```python
from build123d import *

# Parameters (mm, degrees)
F0_W     = 355.6
F0_H     = 203.2
F0_R     = 1.25
F0_R_2   = 20.6375
F1_DEPTH = 2.54


with BuildPart() as f1:
    # F0 (on Front) → F1 (new body)
    with BuildSketch(Plane.XZ):
        with Locations((177.8, 101.6)):
            Rectangle(F0_W, F0_H)
        with BuildLine():
            Line((26.67, 62.23), (41.91, 62.23))
            ThreePointArc((41.91, 62.23), (42.808026, 61.858026), (43.18, 60.96))
            Line((43.18, 60.96), (43.18, 45.72))
            ThreePointArc((43.18, 45.72), (42.808026, 44.821974), (41.91, 44.45))
            Line((41.91, 44.45), (26.67, 44.45))
            ThreePointArc((26.67, 44.45), (25.771974, 44.821974), (25.4, 45.72))
            Line((25.4, 45.72), (25.4, 60.96))
            ThreePointArc((25.4, 60.96), (25.771974, 61.858026), (26.67, 62.23))
        make_face(mode=Mode.SUBTRACT)
        with BuildLine():
            Line((48.26, 62.23), (63.5, 62.23))
            ThreePointArc((63.5, 62.23), (64.398026, 61.858026), (64.77, 60.96))
            Line((64.77, 60.96), (64.77, 45.72))
            ThreePointArc((64.77, 45.72), (64.398026, 44.821974), (63.5, 44.45))
            Line((63.5, 44.45), (48.26, 44.45))
            ThreePointArc((48.26, 44.45), (47.361974, 44.821974), (46.99, 45.72))
            Line((46.99, 45.72), (46.99, 60.96))
            ThreePointArc((46.99, 60.96), (47.361974, 61.858026), (48.26, 62.23))
        make_face(mode=Mode.SUBTRACT)
        with BuildLine():
            Line((69.85, 62.23), (85.09, 62.23))
            ThreePointArc((85.09, 62.23), (85.988026, 61.858026), (86.36, 60.96))
            Line((86.36, 60.96), (86.36, 45.72))
            ThreePointArc((86.36, 45.72), (85.988026, 44.821974), (85.09, 44.45))
            Line((85.09, 44.45), (69.85, 44.45))
            ThreePointArc((69.85, 44.45), (68.951974, 44.821974), (68.58, 45.72))
            Line((68.58, 45.72), (68.58, 60.96))
            ThreePointArc((68.58, 60.96), (68.951974, 61.858026), (69.85, 62.23))
        make_face(mode=Mode.SUBTRACT)
        with Locations((39.624, 105.664)):
            Circle(F0_R, mode=Mode.SUBTRACT)
        with Locations((72.136, 105.664)):
            Circle(F0_R, mode=Mode.SUBTRACT)
        with Locations((55.88, 121.92)):
            Circle(F0_R_2, mode=Mode.SUBTRACT)
        with Locations((39.624, 138.176)):
            Circle(F0_R, mode=Mode.SUBTRACT)
        with Locations((72.136, 138.176)):
            Circle(F0_R, mode=Mode.SUBTRACT)
    extrude(amount=F1_DEPTH)


solid = f1.part
```
Here's how the part is built. I have some questions about the finished solid (model axes, mm). Coordinates: 2 decimals unless noted, no trailing zeros. Order: outer loops, then holes, each group sorted by start corner. A loop starts at its lowest first (then second) coordinate and runs counter-clockwise, first axis right, second up. Notation, with made-up numbers: M 75.5,-37.75 L 102.5,-37.75 A20 cw 102.5,-1.75 Z; hole C 84,39 d6. An arc over 180 degrees is marked long. Answer as a JSON object with one key per item and string values. Group by question number.
(1) Suppose I cut it at A-A, the plane z = 121.92. Please give me the cut outline in (x, y).
(2) Suppose I cut it at B-B, the plane x = 55.88. Please give me the cut outline in (y, z).
(3) I need wall thicknesses on probe 1 along X at (y, z) = (-1.2, 47); probe 2 along Z at (x, y) = (55.88, -2); probe 3 along X at (y, z) = (-1.8, 117). Which ranges of each line are inside material? Lowest first, please.
(4) If we mould it in two halves opening along X, with no side actions, what happens to faces 1 (the face through (175, 0, 103)), 2 (the face through (40.7, -1.3, 135.9))? For each: released by +X, released by -X, zero draft, split by the parting line, or undercut.
(5) For pin 1 (0.8 mm diameter, centred on x = 32, y = -1.5, fed in from -Z), with a flat end and sliding along its axis, tell me the tip position at first contact or that it passes through.
(6) Suppose I cut it at C-C, the plane y = -1.15. State how many separate pieces and enclosed holes the cut face has, then the cut area to 3 significant figures.
Values found:
{
 "1": {"outline": "M 0,-2.54 L 35.24,-2.54 L 35.24,0 L 0,0 Z; M 76.52,-2.54 L 355.6,-2.54 L 355.6,0 L 76.52,0 Z"},
 "2": {"outline": "M -2.54,0 L 0,0 L 0,44.45 L -2.54,44.45 Z; M -2.54,62.23 L 0,62.23 L 0,101.28 L -2.54,101.28 Z; M -2.54,142.56 L 0,142.56 L 0,203.2 L -2.54,203.2 Z"},
 "3": {"probe 1": "x = 0 to 25.4, 43.18 to 46.99, 64.77 to 68.58, 86.36 to 355.6", "probe 2": "z = 0 to 44.45, 62.23 to 101.28, 142.56 to 203.2", "probe 3": "x = 0 to 35.84, 75.92 to 355.6"},
 "4": {"face 1": "zero draft", "face 2": "undercut"},
 "5": {"pin 1": "stops at z = 0"},
 "6": {"separate pieces": "1", "enclosed holes": "8", "area": "70,000 mm^2"}
}
